Check sheet for the modelled part. Datum: model origin and axes. Units: mm. A direction names the side the tool comes from. Round coordinates to 2 decimals unless told otherwise and drop trailing zeros. Order: outer loops, then holes, each group sorted by start corner. A loop starts at its lowest first (then second) coordinate and runs counter-clockwise, first axis right, second up. Notation, with made-up numbers: M 22,58 L 32,58 A18 ccw 32,66 Z; hole C 24,63.5 d11. An arc over 180 degrees is marked long. One line per item, written item: value. Start each with the question number.
(1) Cross-section at D-D, the plane x = 29.5. Enter the section's corners in (y, z), and give its area (3 significant figures).
(2) Access from +Z, -Z, +X, -X, +Y, -Y to the whole of each face (thin tool, end or side, straight path). Record for faces 1 (the face through (-34, 5, -8.357)), 2 (the face through (-34, 5, 20.93)), 3 (the face through (-1, 10, 0)).
(3) Cross-section at C-C, the plane z = -12.5. Enter the section's corners in (x, y).
(4) Release check for a two-part mould opening along X. For faces 4 (the face through (31, 5, -14.336)), 5 (the face through (-39, 5, 25)) record: released by +X, released by -X, zero draft, split by the parting line, or undercut.
(5) Cross-section at B-B, the plane x = 5. Enter the section's corners in (y, z), and give its area (3 significant figures).
(6) Cross-section at A-A, the plane z = -5.5. Enter the section's corners in (x, y), and give its area (3 significant figures).
(7) Thickness scan on L1, parallel to X at y = 3.25, z = 9.5; L2, parallel to Z at x = -28, y = 6.25; L3, parallel to Z at x = 15, y = 8.5. Record the ranges inside material, lowest first.
from build123d import *

# Parameters (mm, degrees)
SKETCH1_W               = 80
SKETCH1_H               = 50
BOSS_EXTRUDE1_DEPTH     = 10
SKETCH2_W               = 8
SKETCH2_H               = 5
CUT_EXTRUDE1_DEPTH      = 49.218253805
CRVPATTERN4_START       = -38
CRVPATTERN4_OUTLINE_W   = 10
CRVPATTERN4_OUTLINE_H   = 4.069772856
CRVPATTERN4_OUTLINE_H_2 = 5
CRVPATTERN4_DEPTH       = 8
CRVPATTERN5_COUNT       = 5
CRVPATTERN5_PITCH       = 9.199623468


# Read off the part's stored shape, not the designer's step: CrvPattern4
with BuildPart() as part:
    # Sketch1 → Boss-Extrude1 (new body)
    with BuildSketch(Plane(origin=(0, 0, 0), x_dir=(1, 0, 0), z_dir=(0, 1, 0))):
        Rectangle(SKETCH1_W, SKETCH1_H)
    extrude(amount=BOSS_EXTRUDE1_DEPTH)

    # Sketch2 → Cut-Extrude1 (cut, through all)
    with BuildSketch(Plane(origin=(0, 10, 0), x_dir=(1, 0, 0), z_dir=(0, 1, 0))):
        with Locations((-34, 20.5)):
            Rectangle(SKETCH2_W, SKETCH2_H)
    cut_extrude1 = extrude(amount=-CUT_EXTRUDE1_DEPTH, mode=Mode.SUBTRACT)

    # CrvPattern4 outline → CrvPattern4 (cut)
    with BuildSketch(Plane.YZ.offset(CRVPATTERN4_START)):
        with Locations((5, 22.965113572)):
            Rectangle(CRVPATTERN4_OUTLINE_W, CRVPATTERN4_OUTLINE_H)
        with Locations((5, 8.786818096)):
            Rectangle(CRVPATTERN4_OUTLINE_W, CRVPATTERN4_OUTLINE_H_2)
        with Locations((5, -5.856590952)):
            Rectangle(CRVPATTERN4_OUTLINE_W, CRVPATTERN4_OUTLINE_H_2)
    extrude(amount=CRVPATTERN4_DEPTH, mode=Mode.SUBTRACT)

    # CrvPattern5: Cut-Extrude1 ×5
    with Locations(*[Vector(0.4999999999066592, 0, 0.866025403838329) * (i * CRVPATTERN5_PITCH) for i in range(1, CRVPATTERN5_COUNT)]):
        add(cut_extrude1, mode=Mode.SUBTRACT)

    # Sketch-Pattern1: Cut-Extrude1 at 7 more places
    with Locations((20.278987, 0, 4.33593), (41.199189, 0, 3.664318), (64.749753, 0, 3.664318), (66.35627, 0, 25.718932), (46.79827, 0, 25.718932), (26.76839, 0, 25.718932), (46.79827, 0, 13.819596)):
        add(cut_extrude1, mode=Mode.SUBTRACT)


solid = part.part
Values found:
1. outline: M 0,-25 L 10,-25 L 10,-19.34 L 0,-19.34 Z; M 0,-14.34 L 10,-14.34 L 10,2.72 L 0,2.72 Z; M 0,7.72 L 10,7.72 L 10,25 L 0,25 Z
1. area: 400 mm^2
2. face 1: +Y, -Y
2. face 2: +Z, +Y, -Y
2. face 3: +Z, -Z, +X, -X, +Y
3. outline: M -40,0 L -33.4,0 L -33.4,10 L -40,10 Z; M -25.4,0 L 40,0 L 40,10 L -25.4,10 Z
4. face 4: undercut
4. face 5: zero draft
5. outline: M 0,-25 L 10,-25 L 10,-19.34 L 0,-19.34 Z; M 0,-14.34 L 10,-14.34 L 10,25 L 0,25 Z
5. area: 450 mm^2
6. outline: M -40,0 L -38,0 L -38,10 L -40,10 Z; M -30,0 L -28.8,0 L -28.8,10 L -30,10 Z; M -20.8,0 L 8.8,0 L 8.8,10 L -20.8,10 Z; M 16.8,0 L 40,0 L 40,10 L 16.8,10 Z
6. area: 560 mm^2
7. L1: -40 to -38, -30 to -19.6, -11.6 to 40
7. L2: -25 to -15.03, -10.03 to -7.07, -2.07 to 25
7. L3: -25 to -9.18, -4.18 to 2.72, 7.72 to 25
